Part model, mm, in its own coordinate system. A direction names the side the tool comes from. Round coordinates to 2 decimals unless told otherwise and drop trailing zeros. Order: outer loops, then holes, each group sorted by start corner. A loop starts at its lowest first (then second) coordinate and runs counter-clockwise, first axis right, second up. Notation, with made-up numbers: (-13.75, -24.75) - (9.25, -24.75) arc R8 ccw to (9.25, -15.75) - close; hole circle Ø8 at (-35.5, -31). An arc over 180 degrees is marked (long way). Return JSON: item names as keys, results as strings. Group by question number.
Item 1: Drop flat-ended pins along their axis: pin 1 (18 mm diameter, centred on x = 60.5, y = -36, fed in from -Z); pin 2 (2.5 mm diameter, centred on x = -1.5, y = -19, fed in from -Z); pin 3 (2 mm diameter, centred on x = 47.5, y = -45.5, fed in from +Z). Give the stop position or say it passes through.
Item 2: Two-plate mould, pull along X, no slides. Class faces 1 (the face through (-5, -30, 9)), 2 (the face through (9, -30, 17.5)), 3 (the face through (17, -30, -10)): released by +X, released by -X, zero draft, split by the parting line, or undercut.
Item 3: Probe probe 1 along X at (y, z) = (-55, 4); probe 2 along Z at (x, y) = (15.5, -38); probe 3 along X at (y, z) = (-17, -13). List the from-to ranges inside material, lowest first.
Item 4: Saw through at A-A on z = 8. List the corners of the cut face in (x, y).
Item 5: Tool access for faces 4 (the face through (69, -30, -18.402)), 5 (the face through (114, -30, 5)), 6 (the face through (66.4, -29.6, -2.5)): list every direction of +Z, -Z, +X, -X, +Y, -Y with a clear straight run to the whole face (end or side of a thin tool).
Item 6: Saw through at C-C on z = -10. List the corners of the cut face in (x, y).
Item 7: Saw through at B-B on y = -27. List the corners of the cut face in (x, z), and give its area (3 significant figures).
Item 8: Saw through at D-D on x = 3. List the corners of the cut face in (y, z), and give its area (3 significant figures).
```python
from build123d import *

# Parameters (mm, degrees)
F1_DEPTH = 60
F3_DEPTH = 90
F5_DEPTH = 5


with BuildPart() as f1:
    # F0 (on Front) → F1 (new body)
    with BuildSketch(Plane.XZ):
        Polygon((-5, 0), (0, 0), (0, 12.5), (17, 12.5), (17, -32.5), (22, -32.5), (22, 17.5), (-5, 17.5), align=None)
    extrude(amount=F1_DEPTH)

    # F2 (on face) → F3 (join)
    with BuildSketch(Plane.YZ.offset(22)):
        with BuildLine():
            Line((-60, -18.402278), (0, -18.402278))
            Line((0, -18.402278), (0, -11.402278))
            ThreePointArc((0, -11.402278), (-30, -2.5), (-60, -11.402278))
            Line((-60, -11.402278), (-60, -18.402278))
        make_face()
    extrude(amount=F3_DEPTH)

    # F4 (on face) → F5 (join)
    with BuildSketch(Plane.YZ.offset(112)):
        with BuildLine():
            ThreePointArc((-60, -11.402278), (-30, -2.5), (0, -11.402278))
            Line((0, -11.402278), (0, -2.67072))
            ThreePointArc((0, -2.67072), (-30, 5), (-60, -2.67072))
            Line((-60, -2.67072), (-60, -11.402278))
        make_face()
        with BuildLine():
            Line((-60, -18.402278), (0, -18.402278))
            Line((0, -18.402278), (0, -11.402278))
            ThreePointArc((0, -11.402278), (-30, -2.5), (-60, -11.402278))
            Line((-60, -11.402278), (-60, -18.402278))
        make_face()
    extrude(amount=F5_DEPTH)


solid = f1.part
```
Filled in:
{
 "1": {"pin 1": "stops at z = -18.4", "pin 2": "stops at z = 0", "pin 3": "stops at z = -4.45"},
 "2": {"face 1": "released by -X", "face 2": "zero draft", "face 3": "undercut"},
 "3": {"probe 1": "x = -5 to 0, 17 to 22", "probe 2": "z = 12.5 to 17.5", "probe 3": "x = 17 to 117"},
 "4": {"outline": "(-5, -60) - (0, -60) - (0, 0) - (-5, 0) - close; (17, -60) - (22, -60) - (22, 0) - (17, 0) - close"},
 "5": {"face 4": "-Z, +X, +Y, -Y", "face 5": "+Z, +X", "face 6": "+Z"},
 "6": {"outline": "(17, -60) - (22, -60) - (22, -57.73) - (112, -57.73) - (112, -60) - (117, -60) - (117, 0) - (112, 0) - (112, -2.27) - (22, -2.27) - (22, 0) - (17, 0) - close"},
 "7": {"outline": "(-5, 0) - (0, 0) - (0, 12.5) - (17, 12.5) - (17, -32.5) - (22, -32.5) - (22, -18.4) - (117, -18.4) - (117, 4.93) - (112, 4.93) - (112, -2.58) - (22, -2.58) - (22, 17.5) - (-5, 17.5) - close", "area": "1,960 mm^2"},
 "8": {"outline": "(-60, 12.5) - (0, 12.5) - (0, 17.5) - (-60, 17.5) - close", "area": "300 mm^2"}
}
